from build123d import *

# Parameters (mm, degrees)
SKETCH1_R           = 3
SKETCH1_R_2         = 2.25
BOSS_EXTRUDE1_DEPTH = 5


with BuildPart() as part:
    # Sketch1 → Boss-Extrude1 (new body)
    with BuildSketch(Plane.XY):
        Polygon((-13, 7.25), (-13, -7.25), (-10, -7.25), (-10, -5.25), (10, -5.25), (10, -7.25), (13, -7.25), (13, 7.25), (10, 7.25), (10, 5.25), (-10, 5.25), (-10, 7.25), align=None)
        with Locations((-9.3, 0)):
            Circle(SKETCH1_R, mode=Mode.SUBTRACT)
        Circle(SKETCH1_R_2, mode=Mode.SUBTRACT)
        with Locations((9.3, 0)):
            Circle(SKETCH1_R, mode=Mode.SUBTRACT)
    extrude(amount=BOSS_EXTRUDE1_DEPTH)


solid = part.part
Read the model definition and answer for the solid it produces. Units are mm, in the model's axes. A direction names the side the tool comes from. Round coordinates to 2 decimals unless told otherwise and drop trailing zeros. Write each loop counter-clockwise with the first axis right and the second up, starting at its lowest first coordinate (ties: lowest second). Pieces come first, ordered by that corner, then holes.
Q1. Flat-ended cylindrical pins translate along their axes: P1, Ø5.5, axis at x = 9.3, y = 0, coming from the +Z side; P2, Ø2, axis at x = 4.5, y = 5.5, coming from the -Z side; P3, Ø3, axis at x = -4, z = 2.5, coming from the +Y side. Find the tip coordinate at first contact, or state that the pin passes through.
Values:
P1: passes through
P2: stops at z = 0
P3: stops at y = 5.25
Q2. The mould has two halves that part along X. Classify faces 4 (the face through (0, -5.25, 2)), 5 (the face through (11, -7.25, 2)), 6 (the face through (-6.53, -1.15, 2.46)), 7 (the face through (-13, 0, 2)): released by +X, released by -X, zero draft, split by the parting line, or undercut.
Values:
face 4: undercut
face 5: zero draft
face 6: undercut
face 7: released by -X
Q3. Find section A-A on x = 9.3. Determine the outline of the cut face in (y, z).
Values:
outline: (-5.25, 0) - (-3, 0) - (-3, 5) - (-5.25, 5) - close; (3, 0) - (5.25, 0) - (5.25, 5) - (3, 5) - close
Q4. Find section C-C on y = 0. Determine the outline of the cut face in (x, z), and give its area (3 significant figures).
Values:
outline: (-13, 0) - (-12.3, 0) - (-12.3, 5) - (-13, 5) - close; (-6.3, 0) - (-2.25, 0) - (-2.25, 5) - (-6.3, 5) - close; (2.25, 0) - (6.3, 0) - (6.3, 5) - (2.25, 5) - close; (12.3, 0) - (13, 0) - (13, 5) - (12.3, 5) - close
area: 47.5 mm2
Q5. Straight lines are drawn through the part: line 1 (Y direction, x = -9.3, z = 1.4); line 2 (X direction, y = 0.5, z = 2.15); line 3 (X direction, y = 1.25, z = 4.6). For each, find the intervals that lie inside material, in ascending order.
Values:
line 1: y = -5.25 to -3, 3 to 5.25
line 2: x = -13 to -12.26, -6.34 to -2.19, 2.19 to 6.34, 12.26 to 13
line 3: x = -13 to -12.03, -6.57 to -1.87, 1.87 to 6.57, 12.03 to 13
Q6. A tool of negligible diameter and unlimited length cuts with its end or side. For faces 1 (the face through (-10, -6, 2)), 2 (the face through (-10, 6, 2)), 3 (the face through (-0.29, 2.23, 2.46)), from which of +Z, -Z, +X, -X, +Y, -Y can it reach the whole face along a straight path? Write none if from no direction.
Values:
face 1: +Z, -Z, -Y
face 2: +Z, -Z, +Y
face 3: +Z, -Z
Q7. Find section B-B on y = 5.5. Determine the outline of the cut face in (x, z), and give its area (3 significant figures).
Values:
outline: (-13, 0) - (-10, 0) - (-10, 5) - (-13, 5) - close; (10, 0) - (13, 0) - (13, 5) - (10, 5) - close
area: 30.0 mm2
Q8. Find section D-D on z = 2.2. Determine the outline of the cut face in (x, y), and give its area (3 significant figures).
Values:
outline: (-13, -7.25) - (-10, -7.25) - (-10, -5.25) - (10, -5.25) - (10, -7.25) - (13, -7.25) - (13, 7.25) - (10, 7.25) - (10, 5.25) - (-10, 5.25) - (-10, 7.25) - (-13, 7.25) - close; hole circle Ø6 at (-9.3, 0); hole circle Ø4.5 at (0, 0); hole circle Ø6 at (9.3, 0)
area: 225 mm2
